```python
from build123d import *

# Parameters (mm, degrees)
BOSS_EXTRUDE1_DEPTH      = 10.35
BOSS_EXTRUDE2_DEPTH      = 2
BOSS_EXTRUDE2_DEPTH_BACK = 2
CHAMFER1_SIZE            = 0.5


with BuildPart() as part:
    # Sketch2 → Boss-Extrude1 (new body)
    with BuildSketch(Plane.XY):
        with BuildLine():
            Line((-2, 2.25), (2, 2.25))
            ThreePointArc((2, 2.25), (4.25, 0), (2, -2.25))
            Line((2, -2.25), (-2, -2.25))
            ThreePointArc((-2, -2.25), (-4.25, 0), (-2, 2.25))
        make_face()
    extrude(amount=BOSS_EXTRUDE1_DEPTH)

    # Sketch5 → Boss-Extrude2 (add, two sides)
    with BuildSketch(Plane(origin=(0, 0, 0), x_dir=(0, 0, -1), z_dir=(1, 0, 0))) as boss_extrude2_sk:
        Polygon((-1.647938398, 2.25), (-0.754123204, 3), (0, 3), (0, 2.25), align=None)
        Polygon((-1.647938398, -2.25), (0, -2.25), (0, -3), (-0.754123204, -3), align=None)
    extrude(amount=BOSS_EXTRUDE2_DEPTH)
    extrude(boss_extrude2_sk.sketch, amount=-BOSS_EXTRUDE2_DEPTH_BACK)

    # Chamfer1
    chamfer1_edges = [part.edges().sort_by_distance(p)[0] for p in [
        (4.25, 0, 10.35),
        (0, 2.25, 10.35),
        (-4.25, 0, 10.35),
        (0, -2.25, 10.35),
    ]]
    chamfer(chamfer1_edges, length=CHAMFER1_SIZE)


solid = part.part
```
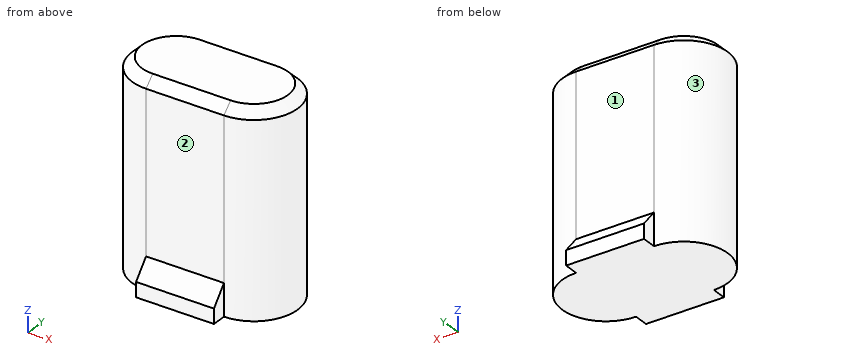
Geometry: final body of the model. Coordinates: model frame, mm. Face numbers are marked on the shaded views. A direction names the side the tool comes from. Coordinates: 2 decimals unless noted, no trailing zeros. Order: outer loops, then holes, each group sorted by start corner. A loop starts at its lowest first (then second) coordinate and runs counter-clockwise, first axis right, second up. Notation, with made-up numbers: (80, 70.5) -> (105, 70.5) arc R16 cw to (105, 79.5) -> close; hole circle Ø10 at (39, -29). An arc over 180 degrees is marked (long way). Answer in a Markdown table with one row per item.
Item 1: Section B-B on z = 9.5. Output: boundary loops of the cut face in (x, y), plus the area to 3 significant figures.
Return value:
| item | result |
|---|---|
| outline | (-2, -2.25) -> (2, -2.25) arc R2.25 ccw to (2, 2.25) -> (-2, 2.25) arc R2.25 ccw to start |
| area | 33.9 mm² |
Item 2: Section A-A on x = -0.5. Output: boundary loops of the cut face in (y, z).
Return value:
| item | result |
|---|---|
| outline | (-3, 0) -> (3, 0) -> (3, 0.75) -> (2.25, 1.65) -> (2.25, 9.85) -> (1.75, 10.35) -> (-1.75, 10.35) -> (-2.25, 9.85) -> (-2.25, 1.65) -> (-3, 0.75) -> close |
Item 3: Section C-C on y = 2.6. Output: boundary loops of the cut face in (x, z), plus the area to 3 significant figures.
Return value:
| item | result |
|---|---|
| outline | (-2, 0) -> (2, 0) -> (2, 1.23) -> (-2, 1.23) -> close |
| area | 4.92 mm² |
Item 4: Ray query, L1, parallel to Y at x = -1.25, z = 9.5; L2, parallel to Y at x = -4, z = 9; L3, parallel to X at y = -0.85, z = 10.25. Return the intervals inside material, ascending.
Return value:
| item | result |
|---|---|
| L1 | y = -2.25 to 2.25 |
| L2 | y = -1.03 to 1.03 |
| L3 | x = -3.64 to 3.64 |
Item 5: Contact query for flat-ended pins moving along their axis: P1, Ø1.5, axis at x = 2.5, y = -1, coming from the -Z side; P2, Ø2, axis at x = 0.5, z = 7, coming from the +Y side; P3, Ø3, axis at x = 0, z = 4, coming from the -Y side. Output: stop coordinate, or through.
Return value:
| item | result |
|---|---|
| P1 | stops at z = 0 |
| P2 | stops at y = 2.25 |
| P3 | stops at y = -2.25 |
Item 6: Access query for the marked faces 1, 2 and 3. Directions: +Z, -Z, +X, -X, +Y, -Y. A direction counts if a zero-diameter tool reaches every point of the face in a straight line with its end or side. Return the directions, or none.
Return value:
| item | result |
|---|---|
| face 1 | +Z, +X, -X, +Y |
| face 2 | +Z, +X, -X, -Y |
| face 3 | +Z, -Z, -X |
